Verification items for the finished model (mm, model axes). A direction names the side the tool comes from. Give positions to 0.01 mm unless a question says otherwise; leave off trailing zeros. Loops run counter-clockwise (first coordinate to the right, second up) from the corner with the lowest first, then second, coordinate; pieces in that order, holes last. Notation, with made-up numbers: (33.5, 31) -> (52.5, 31) arc R21 ccw to (52.5, 66) -> close; hole circle Ø6 at (58.25, -11.75). An arc over 180 degrees is marked (long way). Answer in a Markdown table with one row per item. Add a question column.
Q1. Section check A-A on z = 11. Enter the section's corners in (x, y), and give its area (3 significant figures).
Q2. Section check C-C on z = 3. Enter the section's corners in (x, y).
Q3. Section check B-B on x = 2. Enter the section's corners in (y, z).
Q4. Set-up check for faces 1 (the face through (12.7, 7, 15)), 2 (the face through (-5.48, 16.15, 39.6)): record each of +Z, -Z, +X, -X, +Y, -Y from which the full face is reachable in a straight line by a thin tool's end or side.
Q5. Release check for a two-part mould opening along X. For faces 3 (the face through (0, 7, 15)), 4 (the face through (32.843, 15.76, 38.648)), 5 (the face through (9.53, 13.92, 34.14)), 6 (the face through (17.615, 14.087, 34.545)) record: pulls with the +X half, pulls with the -X half, needs draft (parallel to the pull), parting line crosses it, or undercut.
Q6. Material ranges on probe 1 along X at (y, z) = (4, 15); probe 2 along X at (y, z) = (25, 31); probe 3 along X at (y, z) = (18, 30), recorded low to high.
Q7. Section check D-D on x = 10. Enter the section's corners in (y, z), and give its area (3 significant figures).
Q8. Gauge pin test, flat ends, axial feed: P1, Ø5, axis at x = 2.5, y = 24.5, coming from the -Z side; P2, Ø5, axis at y = 12.5, z = 11.5, coming from the +X side; P3, Ø3, axis at x = 27, y = 8, coming from the +Z side. Record the tip position at first contact, or that the pin passes through.
```python
from build123d import *

# Parameters (mm, degrees)
F1_ANGLE = 45


with BuildPart() as f1:
    # F0 (on Front) → F1 (revolve)
    with BuildSketch(Plane.XZ):
        Polygon((0, 25.4), (0, 0), (12.7, 0), (12.7, 24.531622), (42.501195, 41.73735), (23.451195, 41.73735), (11.940171, 32.998289), (5.861538, 42.767522), (-16.499144, 42.767522), align=None)
    revolve(axis=Axis((6.35, 0, 0), (-1, 0, 0)), revolution_arc=F1_ANGLE)


solid = f1.part
```
Taken from the geometry:
| question | item | result |
|---|---|---|
| 1 | outline | (0, 0) -> (12.7, 0) -> (12.7, 11) -> (0, 11) -> close |
| 1 | area | 140 mm² |
| 2 | outline | (0, 0) -> (12.7, 0) -> (12.7, 3) -> (0, 3) -> close |
| 3 | outline | (0, 0) -> (30.24, 30.24) arc R42.77 ccw to (0, 42.77) -> close |
| 4 | face 1 | -Z, +X, -Y |
| 4 | face 2 | +Z, +X, -X, +Y |
| 5 | face 3 | pulls with the -X half |
| 5 | face 4 | needs draft |
| 5 | face 5 | undercut |
| 5 | face 6 | undercut |
| 6 | probe 1 | x = 0 to 12.7 |
| 6 | probe 2 | x = -13.7 to 7.69, 20.93 to 39.19 |
| 6 | probe 3 | x = -9.11 to 10.7, 14.56 to 30.81 |
| 7 | outline | (0, 0) -> (25.54, 25.54) arc R36.12 ccw to (0, 36.12) -> close |
| 7 | area | 512 mm² |
| 8 | P1 | stops at z = 22 |
| 8 | P2 | stops at x = 12.7 |
| 8 | P3 | stops at z = 41.23 |
